Could you check a few things on this drawing? It's one solid part, dimensions in mm from its lowest x, y, z. Round coordinates to 2 decimals unless told otherwise and drop trailing zeros. Write each loop counter-clockwise with the first axis right and the second up, starting at its lowest first coordinate (ties: lowest second). Pieces come first, ordered by that corner, then holes. Notation, with made-up numbers: M -36,22 L 4,22 A23 cw 4,53 Z; hole C 78.25,87.25 d6. An arc over 180 degrees is marked long. One line per item, written item: value. Start each with the question number.
(1) I want a section at B-B on y = 17.5. Please give me the cut outline in (x, z), and give its area (3 significant figures).
(2) I want a section at D-D on y = 6. Please give me the cut outline in (x, z).
(3) I want a section at C-C on x = 40. Please give me the cut outline in (y, z), and give its area (3 significant figures).
(4) I'm going to push a flat-ended pin straight in: pin 1 Ø1.5 at (y, z) = (16, 2.5) entering from -X. Where does the tip first touch, or does it pass through?
(5) If I drill on L1, parallel to Y at x = 40, z = 2.65; L2, parallel to X at y = 15.5, z = 4.1; L3, parallel to X at y = 5.5, z = 2.35, over which ranges is the centre line in solid material (lowest first)?
(6) I want a section at A-A on z = 0.9. Count the separate pieces of the cut face and the enclosed holes in it, and give its area (3 significant figures).
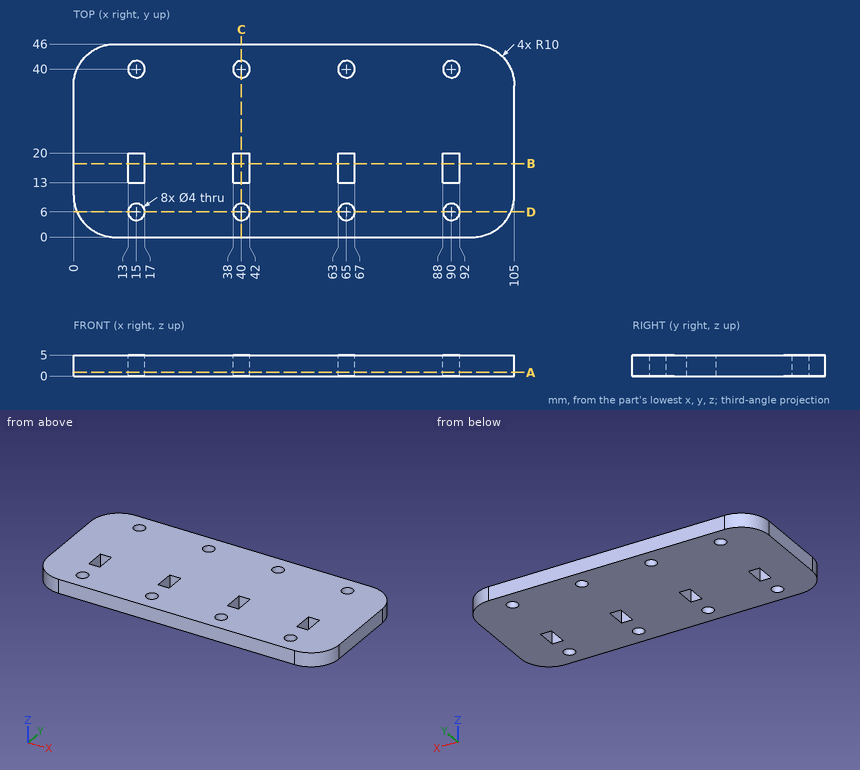
Found:
1. outline: M 0,0 L 13,0 L 13,5 L 0,5 Z; M 17,0 L 38,0 L 38,5 L 17,5 Z; M 42,0 L 63,0 L 63,5 L 42,5 Z; M 67,0 L 88,0 L 88,5 L 67,5 Z; M 92,0 L 105,0 L 105,5 L 92,5 Z
1. area: 445 mm²
2. outline: M 0.83,0 L 13,0 L 13,5 L 0.83,5 Z; M 17,0 L 38,0 L 38,5 L 17,5 Z; M 42,0 L 63,0 L 63,5 L 42,5 Z; M 67,0 L 88,0 L 88,5 L 67,5 Z; M 92,0 L 104.17,0 L 104.17,5 L 92,5 Z
3. outline: M 0,0 L 4,0 L 4,5 L 0,5 Z; M 8,0 L 13,0 L 13,5 L 8,5 Z; M 20,0 L 38,0 L 38,5 L 20,5 Z; M 42,0 L 46,0 L 46,5 L 42,5 Z
3. area: 155 mm²
4. pin 1: stops at x = 0
5. L1: y = 0 to 4, 8 to 13, 20 to 38, 42 to 46
5. L2: x = 0 to 13, 17 to 38, 42 to 63, 67 to 88, 92 to 105
5. L3: x = 1.07 to 13.06, 16.94 to 38.06, 41.94 to 63.06, 66.94 to 88.06, 91.94 to 103.93
6. separate pieces: 1
6. enclosed holes: 12
6. area: 4,530 mm²
